```python
from build123d import *

# Parameters (mm, degrees)
F0_R     = 2.5
F0_R_2   = 1.075
F0_R_3   = 3.125
F0_R_4   = 1.625
F0_R_5   = 7.5
F1_DEPTH = 3


with BuildPart() as f1:
    # F0 (on Top) → F1 (new body)
    with BuildSketch(Plane.XY):
        with BuildLine():
            Line((0.569565, 31), (-0.569565, 31))
            ThreePointArc((-0.569565, 31), (-8.926702, 32.829742), (-15.754697, 37.984173))
            Line((-15.754697, 37.984173), (-46.49461, 73.847404))
            ThreePointArc((-46.49461, 73.847404), (-49.125284, 77.77494), (-50.760679, 82.210193))
            ThreePointArc((-50.760679, 82.210193), (-50.962024, 82.926601), (-51.218827, 83.625051))
            ThreePointArc((-51.218827, 83.625051), (-55.064832, 84.230144), (-55.074594, 88.123446))
            ThreePointArc((-55.074594, 88.123446), (-56.708639, 88.911619), (-58.462718, 89.374794))
            ThreePointArc((-58.462718, 89.374794), (-61.287272, 90.284092), (-63.720645, 91.982215))
            ThreePointArc((-63.720645, 91.982215), (-70.412662, 92.148106), (-71.272207, 85.509447))
            ThreePointArc((-71.272207, 85.509447), (-69.966225, 82.844989), (-69.499616, 79.914595))
            ThreePointArc((-69.499616, 79.914595), (-69.310161, 78.110315), (-68.781173, 76.374949))
            ThreePointArc((-68.781173, 76.374949), (-64.935168, 75.769856), (-64.925406, 71.876554))
            ThreePointArc((-64.925406, 71.876554), (-64.274449, 71.515951), (-63.597263, 71.207407))
            ThreePointArc((-63.597263, 71.207407), (-59.464309, 68.912919), (-55.985318, 65.712512))
            Line((-55.985318, 65.712512), (-33.129578, 39.047482))
            ThreePointArc((-33.129578, 39.047482), (-24.280666, 25.301606), (-19.470554, 9.677419))
            ThreePointArc((-19.470554, 9.677419), (-18.791892, 8.475998), (-17.49674, 8))
            Line((-17.49674, 8), (-16, 8))
            ThreePointArc((-16, 8), (-15.292893, 7.707107), (-15, 7))
            Line((-15, 7), (-15, -7))
            ThreePointArc((-15, -7), (-15.292893, -7.707107), (-16, -8))
            Line((-16, -8), (-17.49674, -8))
            ThreePointArc((-17.49674, -8), (-18.791892, -8.475998), (-19.470554, -9.677419))
            ThreePointArc((-19.470554, -9.677419), (-24.280666, -25.301606), (-33.129578, -39.047482))
            Line((-33.129578, -39.047482), (-55.985318, -65.712512))
            ThreePointArc((-55.985318, -65.712512), (-59.464309, -68.912919), (-63.597263, -71.207407))
            ThreePointArc((-63.597263, -71.207407), (-64.274449, -71.515951), (-64.925406, -71.876554))
            ThreePointArc((-64.925406, -71.876554), (-64.935168, -75.769856), (-68.781173, -76.374949))
            ThreePointArc((-68.781173, -76.374949), (-69.310161, -78.110315), (-69.499616, -79.914595))
            ThreePointArc((-69.499616, -79.914595), (-69.966225, -82.844989), (-71.272207, -85.509447))
            ThreePointArc((-71.272207, -85.509447), (-70.412662, -92.148106), (-63.720645, -91.982215))
            ThreePointArc((-63.720645, -91.982215), (-61.287272, -90.284092), (-58.462718, -89.374794))
            ThreePointArc((-58.462718, -89.374794), (-56.708639, -88.911619), (-55.074594, -88.123446))
            ThreePointArc((-55.074594, -88.123446), (-55.064832, -84.230144), (-51.218827, -83.625051))
            ThreePointArc((-51.218827, -83.625051), (-50.962024, -82.926601), (-50.760679, -82.210193))
            ThreePointArc((-50.760679, -82.210193), (-49.125284, -77.77494), (-46.49461, -73.847404))
            Line((-46.49461, -73.847404), (-15.754697, -37.984173))
            ThreePointArc((-15.754697, -37.984173), (-8.926702, -32.829742), (-0.569565, -31))
            Line((-0.569565, -31), (0.569565, -31))
            ThreePointArc((0.569565, -31), (8.926702, -32.829742), (15.754697, -37.984173))
            Line((15.754697, -37.984173), (46.49461, -73.847404))
            ThreePointArc((46.49461, -73.847404), (49.125284, -77.77494), (50.760679, -82.210193))
            ThreePointArc((50.760679, -82.210193), (50.962024, -82.926601), (51.218827, -83.625051))
            ThreePointArc((51.218827, -83.625051), (55.064832, -84.230144), (55.074594, -88.123446))
            ThreePointArc((55.074594, -88.123446), (56.708639, -88.911619), (58.462718, -89.374794))
            ThreePointArc((58.462718, -89.374794), (61.287272, -90.284092), (63.720645, -91.982215))
            ThreePointArc((63.720645, -91.982215), (70.412662, -92.148106), (71.272207, -85.509447))
            ThreePointArc((71.272207, -85.509447), (69.966225, -82.844989), (69.499616, -79.914595))
            ThreePointArc((69.499616, -79.914595), (69.310161, -78.110315), (68.781173, -76.374949))
            ThreePointArc((68.781173, -76.374949), (64.935168, -75.769856), (64.925406, -71.876554))
            ThreePointArc((64.925406, -71.876554), (64.274449, -71.515951), (63.597263, -71.207407))
            ThreePointArc((63.597263, -71.207407), (59.464309, -68.912919), (55.985318, -65.712512))
            Line((55.985318, -65.712512), (33.129578, -39.047482))
            ThreePointArc((33.129578, -39.047482), (24.280666, -25.301606), (19.470554, -9.677419))
            ThreePointArc((19.470554, -9.677419), (18.791892, -8.475998), (17.49674, -8))
            Line((17.49674, -8), (16, -8))
            ThreePointArc((16, -8), (15.292893, -7.707107), (15, -7))
            Line((15, -7), (15, 7))
            ThreePointArc((15, 7), (15.292893, 7.707107), (16, 8))
            Line((16, 8), (17.49674, 8))
            ThreePointArc((17.49674, 8), (18.791892, 8.475998), (19.470554, 9.677419))
            ThreePointArc((19.470554, 9.677419), (24.280666, 25.301606), (33.129578, 39.047482))
            Line((33.129578, 39.047482), (55.985318, 65.712512))
            ThreePointArc((55.985318, 65.712512), (59.464309, 68.912919), (63.597263, 71.207407))
            ThreePointArc((63.597263, 71.207407), (64.274449, 71.515951), (64.925406, 71.876554))
            ThreePointArc((64.925406, 71.876554), (64.935168, 75.769856), (68.781173, 76.374949))
            ThreePointArc((68.781173, 76.374949), (69.310161, 78.110315), (69.499616, 79.914595))
            ThreePointArc((69.499616, 79.914595), (69.966225, 82.844989), (71.272207, 85.509447))
            ThreePointArc((71.272207, 85.509447), (70.412662, 92.148106), (63.720645, 91.982215))
            ThreePointArc((63.720645, 91.982215), (61.287272, 90.284092), (58.462718, 89.374794))
            ThreePointArc((58.462718, 89.374794), (56.708639, 88.911619), (55.074594, 88.123446))
            ThreePointArc((55.074594, 88.123446), (55.064832, 84.230144), (51.218827, 83.625051))
            ThreePointArc((51.218827, 83.625051), (50.962024, 82.926601), (50.760679, 82.210193))
            ThreePointArc((50.760679, 82.210193), (49.125284, 77.77494), (46.49461, 73.847404))
            Line((46.49461, 73.847404), (15.754697, 37.984173))
            ThreePointArc((15.754697, 37.984173), (8.926702, 32.829742), (0.569565, 31))
        make_face()
        with Locations((-67.158705, -88.351823)):
            Circle(F0_R, mode=Mode.SUBTRACT)
        with Locations((-59.539821, -85.982327)):
            Circle(F0_R_2, mode=Mode.SUBTRACT)
        with Locations((-65.982327, -80.460179)):
            Circle(F0_R_2, mode=Mode.SUBTRACT)
        with Locations((-60, -80)):
            Circle(F0_R_3, mode=Mode.SUBTRACT)
        with Locations((-60.460179, -74.017673)):
            Circle(F0_R_2, mode=Mode.SUBTRACT)
        with Locations((-54.017673, -79.539821)):
            Circle(F0_R_2, mode=Mode.SUBTRACT)
        with Locations((-15.25, -15.25)):
            Circle(F0_R_4, mode=Mode.SUBTRACT)
        with Locations((-10, -10)):
            Circle(F0_R_4, mode=Mode.SUBTRACT)
        with Locations((54.017673, -79.539821)):
            Circle(F0_R_2, mode=Mode.SUBTRACT)
        with Locations((59.539821, -85.982327)):
            Circle(F0_R_2, mode=Mode.SUBTRACT)
        with Locations((67.158705, -88.351823)):
            Circle(F0_R, mode=Mode.SUBTRACT)
        with Locations((60, -80)):
            Circle(F0_R_3, mode=Mode.SUBTRACT)
        with Locations((60.460179, -74.017673)):
            Circle(F0_R_2, mode=Mode.SUBTRACT)
        with Locations((65.982327, -80.460179)):
            Circle(F0_R_2, mode=Mode.SUBTRACT)
        with Locations((15.25, -15.25)):
            Circle(F0_R_4, mode=Mode.SUBTRACT)
        with Locations((10, -10)):
            Circle(F0_R_4, mode=Mode.SUBTRACT)
        with Locations((-10, 10)):
            Circle(F0_R_4, mode=Mode.SUBTRACT)
        with Locations((-15.25, 15.25)):
            Circle(F0_R_4, mode=Mode.SUBTRACT)
        with Locations((-65.982327, 80.460179)):
            Circle(F0_R_2, mode=Mode.SUBTRACT)
        with Locations((-60.460179, 74.017673)):
            Circle(F0_R_2, mode=Mode.SUBTRACT)
        with Locations((-60, 80)):
            Circle(F0_R_3, mode=Mode.SUBTRACT)
        with Locations((-67.158705, 88.351823)):
            Circle(F0_R, mode=Mode.SUBTRACT)
        with Locations((-59.539821, 85.982327)):
            Circle(F0_R_2, mode=Mode.SUBTRACT)
        with Locations((-54.017673, 79.539821)):
            Circle(F0_R_2, mode=Mode.SUBTRACT)
        Circle(F0_R_5, mode=Mode.SUBTRACT)
        with Locations((10, 10)):
            Circle(F0_R_4, mode=Mode.SUBTRACT)
        with Locations((15.25, 15.25)):
            Circle(F0_R_4, mode=Mode.SUBTRACT)
        with Locations((54.017673, 79.539821)):
            Circle(F0_R_2, mode=Mode.SUBTRACT)
        with Locations((60.460179, 74.017673)):
            Circle(F0_R_2, mode=Mode.SUBTRACT)
        with Locations((60, 80)):
            Circle(F0_R_3, mode=Mode.SUBTRACT)
        with Locations((65.982327, 80.460179)):
            Circle(F0_R_2, mode=Mode.SUBTRACT)
        with Locations((59.539821, 85.982327)):
            Circle(F0_R_2, mode=Mode.SUBTRACT)
        with Locations((67.158705, 88.351823)):
            Circle(F0_R, mode=Mode.SUBTRACT)
    extrude(amount=F1_DEPTH)


solid = f1.part
```
Design review of the part built by this model. Coordinates are the model's own, in mm. A direction names the side the tool comes from. Give positions to 0.01 mm unless a question says otherwise; leave off trailing zeros. Order: outer loops, then holes, each group sorted by start corner. A loop starts at its lowest first (then second) coordinate and runs counter-clockwise, first axis right, second up. Notation, with made-up numbers: M 62,7 L 116,7 A10 ccw 116,18 Z; hole C -14,-38 d2. An arc over 180 degrees is marked long. One line per question, with ' | ' between items. Start each with the question number.
Q1. For pin 1 Ø2.5 at (x, y) = (59.54, 85.98) entering from +Z; pin 2 Ø1 at (y, z) = (19.5, 1.5) entering from -X; pin 3 Ø0.9 at (x, z) = (0, 1.5) entering from -Y; pin 4 Ø1.6 at (x, z) = (16.5, 1.5) entering from -Y, all flat-tipped, find the tip position at first contact; note any pin that passes through.
Q2. The part is to be moulded in two halves that separate along Y. For faces 1 (the face through (-6, -6, 0)), 2 (the face through (-49.155, -77.834, 1.479)), 3 (the face through (44.72, -52.57, 1.48)), say which applies: +Y half, -Y half, draft (parallel to the pull), parting line (faces both ways), or undercut.
Q3. Machinability: for faces 4 (the face through (-44.72, 52.57, 1.48)), 5 (the face through (65.17, -89.87, 1.48)), 6 (the face through (49.095, -77.716, 1.479)), 7 (the face through (-8.82, 32.78, 1.48)), 8 (the face through (24.184, 25.093, 1.479)), which of the approach directions +Z, -Z, +X, -X, +Y, -Y give a long, thin tool a straight path to every point of the face, cutting with its end or side? Answer none if there is none.
Q4. We need section A-A (y = 4.5). Write out the cut boundary in (x, z).
Q5. We need section B-B (x = -28). Write out the cut boundary in (y, z).
Q6. We need section C-C (z = 0.55). State how many separate pieces and enclosed holes the cut face has, plus the area to 3 significant figures.
Q7. For L1, parallel to X at y = 11, z = 1.2; L2, parallel to Y at x = 10.5, z = 2.05; L3, parallel to Y at x = -14, z = 0.5, list the stretches that pass through material, from the lowest coordinate up. Write a range as [from, to].
Q8. We need section D-D (y = 27.5). Write out the cut boundary in (x, z).
Returned:
1) pin 1: z = 3 | pin 2: x = -22.12 | pin 3: y = -31 | pin 4: y = -39.79
2) face 1: draft | face 2: -Y half | face 3: undercut
3) face 4: +Z, -Z, -X | face 5: +Z, -Z | face 6: +Z, -Z, -Y | face 7: +Z, -Z, +Y | face 8: +Z, -Z, +X
4) outline: M -15,0 L -6,0 L -6,3 L -15,3 Z; M 6,0 L 15,0 L 15,3 L 6,3 Z
5) outline: M -52.27,0 L -32.11,0 L -32.11,3 L -52.27,3 Z; M 32.11,0 L 52.27,0 L 52.27,3 L 32.11,3 Z
6) separate pieces: 1 | enclosed holes: 33 | area: 6,190 mm2
7) L1: [-19.7, -11.28], [-8.72, 8.72], [11.28, 19.7] | L2: [-33.64, -11.55], [-8.45, 8.45], [11.55, 33.64] | L3: [-36.18, -16.29], [-14.21, 14.21], [16.29, 36.18]
8) outline: M -25.36,0 L 25.36,0 L 25.36,3 L -25.36,3 Z
